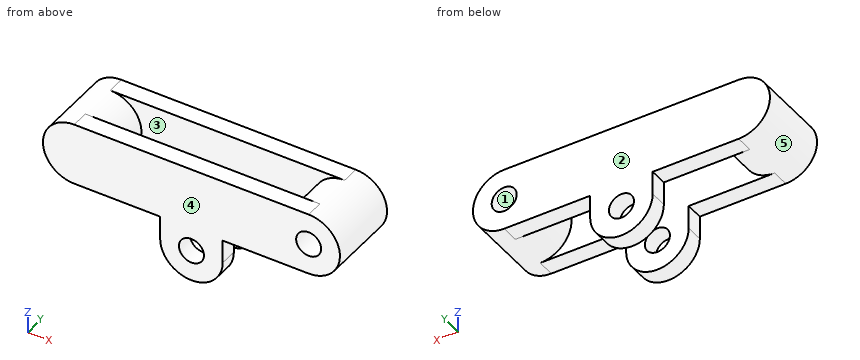
from build123d import *

# Parameters (mm, degrees)
SKETCH1_R               = 1.6
BOSS_EXTRUDE1_DEPTH     = 9.5
CUT_EXTRUDE1_DEPTH      = 2.5
CUT_EXTRUDE1_DEPTH_BACK = 2.5


with BuildPart() as part:
    # Sketch1 → Boss-Extrude1 (new body)
    with BuildSketch(Plane(origin=(0, 0, 0), x_dir=(1, 0, 0), z_dir=(0, 1, 0))):
        with BuildLine():
            Line((0, -4), (-30, -4))
            ThreePointArc((-30, -4), (-34, 0), (-30, 4))
            Line((-30, 4), (-19, 4))
            Line((-19, 4), (-19, 7))
            ThreePointArc((-19, 7), (-15, 11), (-11, 7))
            Line((-11, 7), (-11, 4))
            Line((-11, 4), (0, 4))
            ThreePointArc((0, 4), (4, 0), (0, -4))
        make_face()
        with Locations(Location((0, 0, 0), (0, 0, 270))):
            Circle(SKETCH1_R, mode=Mode.SUBTRACT)
        with Locations(Location((-15, 7, 0), (0, 0, 270))):
            Circle(SKETCH1_R, mode=Mode.SUBTRACT)
    extrude(amount=BOSS_EXTRUDE1_DEPTH)

    # Sketch2 → Cut-Extrude1 (cut, two sides: drawn at the far end of the back side and taken through both)
    with BuildSketch(Plane(origin=(0, 4.75, 0), x_dir=(1, 0, 0), z_dir=(0, 1, 0)).offset(-CUT_EXTRUDE1_DEPTH_BACK)):
        with BuildLine():
            Line((0, 4), (-11, 4))
            Line((-11, 4), (-11, 7))
            ThreePointArc((-11, 7), (-15, 11), (-19, 7))
            Line((-19, 7), (-19, 4))
            Line((-19, 4), (-30, 4))
            ThreePointArc((-30, 4), (-26, 0), (-30, -4))
            Line((-30, -4), (0, -4))
            ThreePointArc((0, -4), (-4, 0), (0, 4))
        make_face()
    extrude(amount=CUT_EXTRUDE1_DEPTH + CUT_EXTRUDE1_DEPTH_BACK, mode=Mode.SUBTRACT)


solid = part.part
Geometry check sheet. Reference: the model listing, model coordinates, mm. Face numbers are marked on the shaded views. A direction names the side the tool comes from. Round coordinates to 2 decimals unless told otherwise and drop trailing zeros. Loops run counter-clockwise (first coordinate to the right, second up) from the corner with the lowest first, then second, coordinate; pieces in that order, holes last. Notation, with made-up numbers: (73.25, -37) - (100.25, -37) arc R21 cw to (100.25, -1) - close; hole circle Ø3 at (36.25, -26). An arc over 180 degrees is marked (long way). One line per question, with ' | ' between items. Start each with the question number.
1. Cross-section at A-A on z = 0. Record the cut outline in (x, y), then the cut area to 3 significant figures.
2. Cross-section at B-B on z = -4.5. Record the cut outline in (x, y), then the cut area to 3 significant figures.
3. Scan lines: line 1 (X direction, y = 3.75, z = 0); line 2 (X direction, y = 1.4, z = -7); line 3 (Z direction, x = -15, y = 8.7). Record each from-to range of solid material in increasing order. Write a range as [from, to].
4. Cross-section at C-C on y = 7.75. Record the cut outline in (x, z), then the cut area to 3 significant figures.
5. Depth check by flat-ended pin: pin 1 (4 mm diameter, centred on y = 2.5, z = -3.5, fed in from +X); pin 2 (2.5 mm diameter, centred on y = 1, z = -6, fed in from -X); pin 3 (3 mm diameter, centred on x = -9, y = 5.5, fed in from -Z); pin 4 (1.1 mm diameter, centred on x = -23, y = 9, fed in from -Z). Enter the tip coordinate at first touch or a pass-through.
6. Cross-section at D-D on x = -8. Record the cut outline in (y, z), then the cut area to 3 significant figures.
7. Draft check along X on the marked faces 1, 2 and 3. Enter one of: released by +X, released by -X, zero draft, split by the parting line, or undercut.
8. Tool access check on the marked faces 4 and 5. Record the directions out of +Z, -Z, +X, -X, +Y, -Y that give a thin tool (end or side, any length) a straight path to the whole face; none if there is none.
Taken from the geometry:
1) outline: (-34, 0) - (-1.6, 0) - (-1.6, 9.5) - (-34, 9.5) - close; (1.6, 0) - (4, 0) - (4, 9.5) - (1.6, 9.5) - close; hole (-26, 2.25) - (-4, 2.25) - (-4, 7.25) - (-26, 7.25) - close | area: 221 mm²
2) outline: (-19, 0) - (-11, 0) - (-11, 2.25) - (-19, 2.25) - close; (-19, 7.25) - (-11, 7.25) - (-11, 9.5) - (-19, 9.5) - close | area: 36.0 mm²
3) line 1: [-34, -26], [-4, -1.6], [1.6, 4] | line 2: [-19, -16.6], [-13.4, -11] | line 3: [-11, -8.6], [-5.4, 4]
4) outline: (-30, -4) - (-19, -4) - (-19, -7) arc R4 ccw to (-11, -7) - (-11, -4) - (0, -4) arc R4 ccw to (0, 4) - (-30, 4) arc R4 ccw to start; hole circle Ø3.2 at (-15, -7); hole circle Ø3.2 at (0, 0) | area: 323 mm²
5) pin 1: x = 3.71 | pin 2: x = -19 | pin 3: through | pin 4: z = -4
6) outline: (0, -4) - (2.25, -4) - (2.25, 4) - (0, 4) - close; (7.25, -4) - (9.5, -4) - (9.5, 4) - (7.25, 4) - close | area: 36.0 mm²
7) face 1: undercut | face 2: zero draft | face 3: undercut
8) face 4: +Z, -Z, +X, -X, -Y | face 5: none
